Here's the drawing with two shaded views (mm, measured from the low corner). I have some questions. A direction names the side the tool comes from. Give positions to 0.01 mm unless a question says otherwise; leave off trailing zeros. Write each loop counter-clockwise with the first axis right and the second up, starting at its lowest first coordinate (ties: lowest second). Pieces come first, ordered by that corner, then holes.
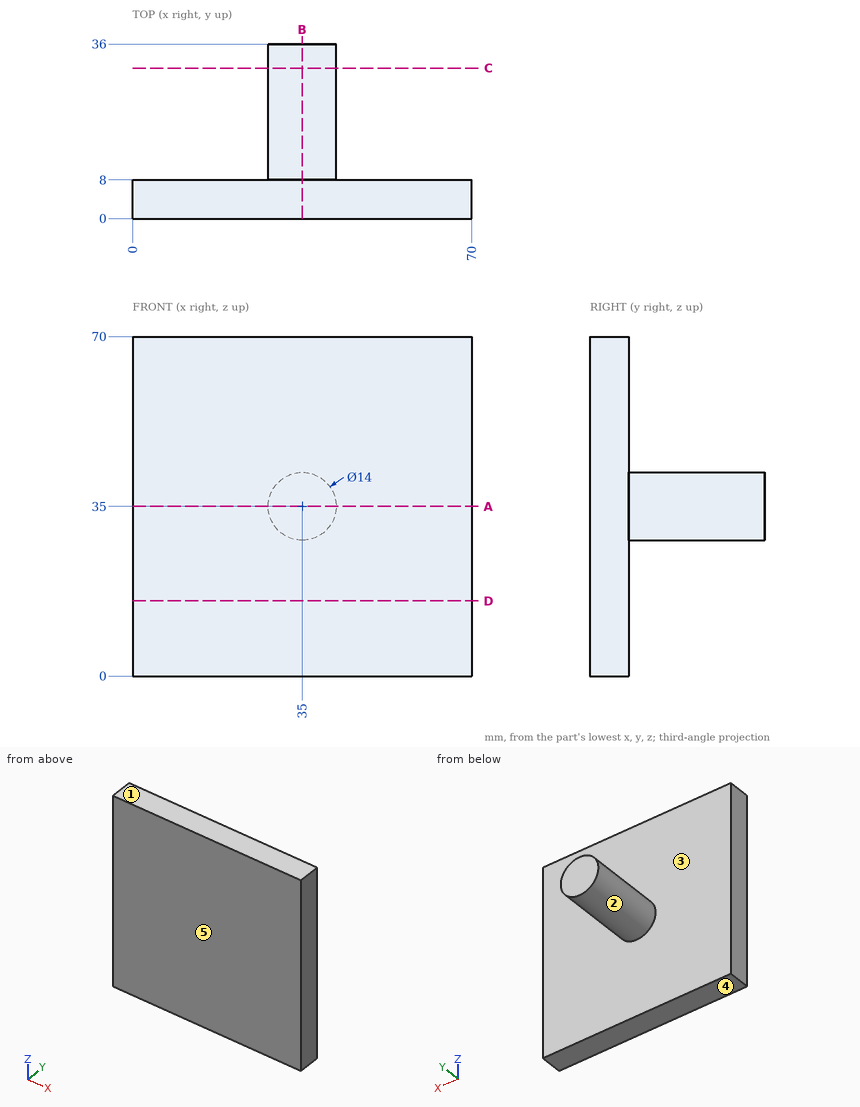
(1) If we mould it in two halves opening along Y, with no side actions, what happens to the marked faces 3, 4 and 5? For each: +Y half, -Y half, draft (parallel to the pull), parting line (faces both ways), or undercut.
Returned:
face 3: +Y half
face 4: draft
face 5: -Y half
(2) Will these pins go through, and if not, where does the flat tip stop? P1, Ø5, axis at x = 19.5, z = 41.5, coming from the +Y side; P2, Ø8, axis at y = 15.5, z = 14.5, coming from the -X side.
Returned:
P1: stops at y = 8
P2: passes through
(3) Imagine slicing it at C-C, the plane y = 31. Write out the boundary of the cut face in (x, z).
Returned:
outline: circle Ø14 at (35, 35)
(4) For the marked faces 1 and 2, which set-ups out of +Z, -Z, +X, -X, +Y, -Y let a thin tool reach every point of the face, with its end or its side?
Returned:
face 1: +Z, +X, -X, +Y, -Y
face 2: +Y
(5) If I drill on L1, parallel to Y at x = 13.5, z = 53; L2, parallel to Z at x = 41, y = 8.5, over which ranges is the centre line in solid material (lowest first)?
Returned:
L1: y = 0 to 8
L2: z = 31.39 to 38.61
(6) Imagine slicing it at B-B, the plane x = 35. Write out the boundary of the cut face in (y, z), plus the area to 3 significant figures.
Returned:
outline: (0, 0) - (8, 0) - (8, 28) - (36, 28) - (36, 42) - (8, 42) - (8, 70) - (0, 70) - close
area: 952 mm2
(7) Imagine slicing it at A-A, the plane z = 35. Write out the boundary of the cut face in (x, y), plus the area to 3 significant figures.
Returned:
outline: (0, 0) - (70, 0) - (70, 8) - (42, 8) - (42, 36) - (28, 36) - (28, 8) - (0, 8) - close
area: 952 mm2
(8) Imagine slicing it at D-D, the plane z = 15.5. Write out the boundary of the cut face in (x, y).
Returned:
outline: (0, 0) - (70, 0) - (70, 8) - (0, 8) - close
